Design review of the part built by this model. Coordinates are the model's own, in mm. Face numbers are marked on the shaded views. Coordinates: 2 decimals unless noted, no trailing zeros. Loops run counter-clockwise (first coordinate to the right, second up) from the corner with the lowest first, then second, coordinate; pieces in that order, holes last. Notation, with made-up numbers: (1, 86) - (52, 86) arc R8 ccw to (52, 101) - close; hole circle Ø4 at (65.25, 48.5). An arc over 180 degrees is marked (long way). Answer in a Markdown table with one row per item. Add a question column.
(1) The part is to be moulded in two halves that separate along Y. For the marked faces 1, 2 and 3, say which applies: released by +Y, released by -Y, zero draft, split by the parting line, or undercut.
(2) We need section D-D, the plane z = 1.25. Write out the cut boundary in (x, y), plus the area to 3 significant figures.
(3) Clearance check with flat-ended pins moving along their axes: pin 1 (1 mm diameter, centred on x = 68.5, y = -47.5, fed in from -Z); pin 2 (8 mm diameter, centred on x = 70.5, y = -38, fed in from +Z). State where each tip first meets the part, or that it passes through.
(4) We need section C-C, the plane x = 66. Write out the cut boundary in (y, z), plus the area to 3 significant figures.
(5) To check wall thickness, follow L1, parallel to Y at x = 64, z = 10.75; L2, parallel to Y at x = 68, z = 5.75; L3, parallel to X at y = -30, z = 1.75. State the ranges of each line that lie inside material, in increasing order. Write a range as [from, to].
(6) We need section B-B, the plane z = 6. Write out the cut boundary in (x, y), plus the area to 3 significant figures.
(7) We need section A-A, the plane x = 75.5. Write out the cut boundary in (y, z), plus the area to 3 significant figures.
Autodesk Inventor part; units mm, degrees
ref_plane "YZ Plane" through (0, 0, 0) normal (1, 0, 0) x (0, 1, 0)
ref_plane "XZ Plane" through (0, 0, 0) normal (0, 1, 0) x (-1, 0, 0)
ref_plane "XY Plane" through (0, 0, 0) normal (0, 0, 1) x (1, 0, 0)
sketch "Sketch1" plane through (0, 0, 0) normal (0, 0, 1) x (1, 0, 0)
  line L0 (0, 0) -> (80, 0)
  line L1 (80, 0) -> (80, -80)
  line L2 (80, -80) -> (0, -80)
  line L3 (0, -80) -> (0, 0)
  dimension "d0" = 80
  dimension "d1" = 80
extrude "Extrusion1" add sketch "Sketch1" along normal blind 15
sketch "Sketch2" plane through (0, 0, 0) normal (0, 0, -1) x (-1, 0, 0)
  line L0 (0, 0) -> (-80, 0)
  circle A0 centre (-60, -40) radius 6.1
  line L1 (-80, 0) -> (-80, -80)
  line L2 (-60, -33.9) -> (-80, -33.9)
  line L3 (-80, -80) -> (-80, 0)
  line L4 (-60, -46.1) -> (-80, -46.1)
  line L5 (-80, -46.1) -> (-80, -33.9)
  dimension "d7" = 40
  dimension "d8" = 20
  dimension "d9" = 12.2
extrude "Extrusion2" cut sketch "Sketch2" against normal through all
sketch "Sketch3" plane through (0, 0, 0) normal (0, 0, -1) x (-1, 0, 0)
  arc A0 (-60, -46.1) -> (-60, -33.9) centre (-60, -40) ccw
  circle A1 centre (-60, -40) radius 8.1
  line L0 (-60, -31.9) -> (-80, -31.9)
  line L1 (-80, -33.9) -> (-80, 0)
  line L2 (-60, -48.1) -> (-80, -48.1)
  line L3 (-80, -48.1) -> (-80, -31.9)
  point P0 (0, 0)
  dimension "d12" = 16.2
extrude "Extrusion3" cut sketch "Sketch3" against normal blind 4
sketch "Sketch4" plane through (0, 0, 15) normal (0, 0, 1) x (1, 0, 0)
  line L0 (80, -31.9) -> (60, -31.9)
  arc A0 (60, -31.9) -> (60, -48.1) centre (60, -40) ccw
  line L1 (60, -48.1) -> (80, -48.1)
  line L2 (80, -46.1) -> (60, -46.1)
  arc A1 (60, -33.9) -> (60, -46.1) centre (60, -40) ccw
  line L3 (60, -33.9) -> (80, -33.9)
  line L4 (80, -33.9) -> (80, -31.9)
  line L5 (80, -33.9) -> (80, 0)
  line L6 (80, -46.1) -> (80, -48.1)
  line L7 (80, -80) -> (80, -46.1)
  point P0 (0, 0)
extrude "Extrusion4" cut sketch "Sketch4" against normal blind 5.5
sketch "Sketch5" plane through (0, 0, 0) normal (0, 0, -1) x (-1, 0, 0)
  arc A0 (-60, -46.1) -> (-60, -33.9) centre (-60, -40) ccw
  line L0 (-80, -31.9) -> (-60, -31.9)
  circle A1 centre (-60, -40) radius 8.1
  line L1 (-60, -31.9) -> (-60, -25)
  line L2 (-72, -25) -> (-72, -55)
  line L3 (-60, -48.1) -> (-60, -55)
  arc A2 (-60, -48.1) -> (-60, -31.9) centre (-60, -40) ccw
  line L4 (-60, -31.9) -> (-60, -31.9)
  line L5 (-60, -31.9) -> (-60, -31.9)
  line L6 (-60, -33.9) -> (-60, -46.1)
  arc A3 (-60, -25) -> (-72, -25) centre (-66, -25) ccw
  arc A4 (-72, -55) -> (-60, -55) centre (-66, -55) ccw
  point P0 (0, 0)
  dimension "d17" = 12
  dimension "d20" = 30
  dimension "d21" = 15
extrude "Extrusion5" cut sketch "Sketch5" against normal blind 4 contours L2 A3 L1 L0 | L0 A1 L3 A4 L2
equation "\"RodDiameter\" = 8"
equation "\"VerticalBearingOD\" = 16"
equation "\"PrintingClearance\" = 0.2"
properties part number "HotendMountCarriage"
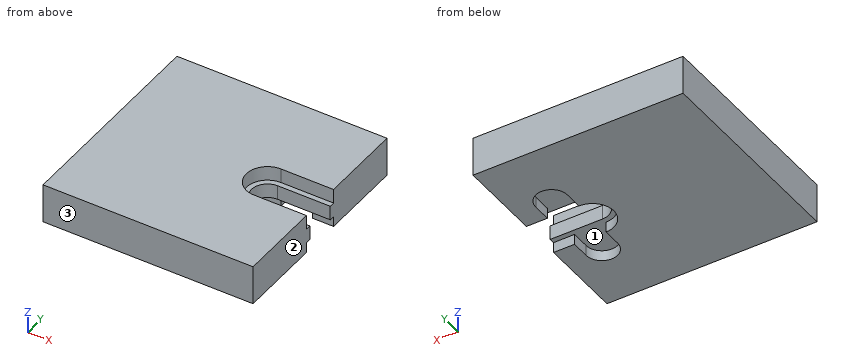
Responses:
| question | item | result |
|---|---|---|
| 1 | face 1 | undercut |
| 1 | face 2 | zero draft |
| 1 | face 3 | released by -Y |
| 2 | outline | (0, -80) - (80, -80) - (80, -48.1) - (72, -48.1) - (72, -55) arc R6 cw to (60, -55) - (60, -48.1) arc R8.1 cw to (60, -31.9) - (60, -25) arc R6 cw to (72, -25) - (72, -31.9) - (80, -31.9) - (80, 0) - (0, 0) - close |
| 2 | area | 5,690 mm2 |
| 3 | pin 1 | stops at z = 4 |
| 3 | pin 2 | passes through |
| 4 | outline | (-80, 0) - (-61, 0) - (-61, 4) - (-46.1, 4) - (-46.1, 9.5) - (-48.1, 9.5) - (-48.1, 15) - (-80, 15) - close; (-33.9, 4) - (-19, 4) - (-19, 0) - (0, 0) - (0, 15) - (-31.9, 15) - (-31.9, 9.5) - (-33.9, 9.5) - close |
| 4 | area | 876 mm2 |
| 5 | L1 | y = [-80, -48.1], [-31.9, 0] |
| 5 | L2 | y = [-80, -46.1], [-33.9, 0] |
| 5 | L3 | x = [0, 60], [72, 80] |
| 6 | outline | (0, -80) - (80, -80) - (80, -46.1) - (60, -46.1) arc R6.1 cw to (60, -33.9) - (80, -33.9) - (80, 0) - (0, 0) - close |
| 6 | area | 6,100 mm2 |
| 7 | outline | (-80, 0) - (-48.1, 0) - (-48.1, 4) - (-46.1, 4) - (-46.1, 9.5) - (-48.1, 9.5) - (-48.1, 15) - (-80, 15) - close; (-33.9, 4) - (-31.9, 4) - (-31.9, 0) - (0, 0) - (0, 15) - (-31.9, 15) - (-31.9, 9.5) - (-33.9, 9.5) - close |
| 7 | area | 979 mm2 |
